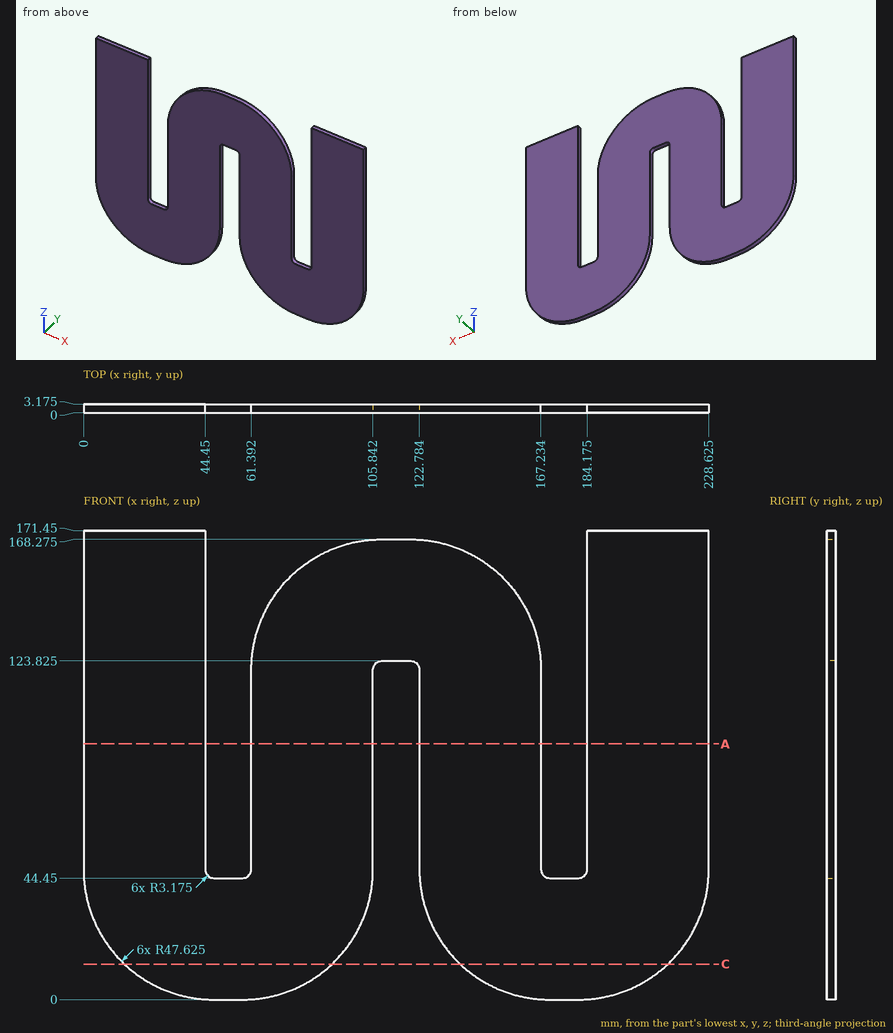
The drawing under review shows one solid part. Ordinate dimensions are in mm from its lowest x, y, z. Coordinates: 2 decimals unless noted, no trailing zeros. Order: outer loops, then holes, each group sorted by start corner. A loop starts at its lowest first (then second) coordinate and runs counter-clockwise, first axis right, second up. Notation, with made-up numbers: (40.5, 74) -> (95.5, 74) arc R16 cw to (95.5, 95) -> close; hole circle Ø9 at (-35.5, 53.25). An arc over 180 degrees is marked (long way). One line per item, written item: value.
1) To check wall thickness, follow probe 1 along X at (y, z) = (1.95, 29); probe 2 along X at (y, z) = (0.25, 25) (1 decimal); probe 3 along Z at (x, y) = (159, 0.9) (1 decimal). State the ranges of each line that lie inside material, in increasing order. Write a range as [from, to].
Output values:
probe 1: x = [3.79, 102.05], [126.58, 224.83]
probe 2: x = [5.7, 100.1], [128.5, 222.9]
probe 3: z = [1.4, 147.4]
2) We need section C-C, the plane z = 13. Give the boundary of the cut face in (x, y) (1 decimal).
Output values:
outline: (14.9, 0) -> (90.9, 0) -> (90.9, 3.2) -> (14.9, 3.2) -> close; (137.7, 0) -> (213.7, 0) -> (213.7, 3.2) -> (137.7, 3.2) -> close
3) Clearance check with flat-ended pins moving along their axes: P1, Ø1.6, axis at x = 52.5, y = 1, coming from the +Z side; P2, Ø5, axis at x = 108.5, z = 60.5, coming from the -Y side; P3, Ø1.6, axis at x = 113, y = 2, coming from the +Z side (3 decimals); P4, Ø1, axis at y = 1.5, z = 34, coming from the -X side (1 decimal). State where each tip first meets the part, or that it passes through.
Output values:
P1: stops at z = 44.45
P2: passes through
P3: stops at z = 168.275
P4: stops at x = 1.8
4) We need section A-A, the plane z = 93.5. Count the separate pieces of the cut face and the enclosed holes in it.
Output values:
separate pieces: 4
enclosed holes: 0
